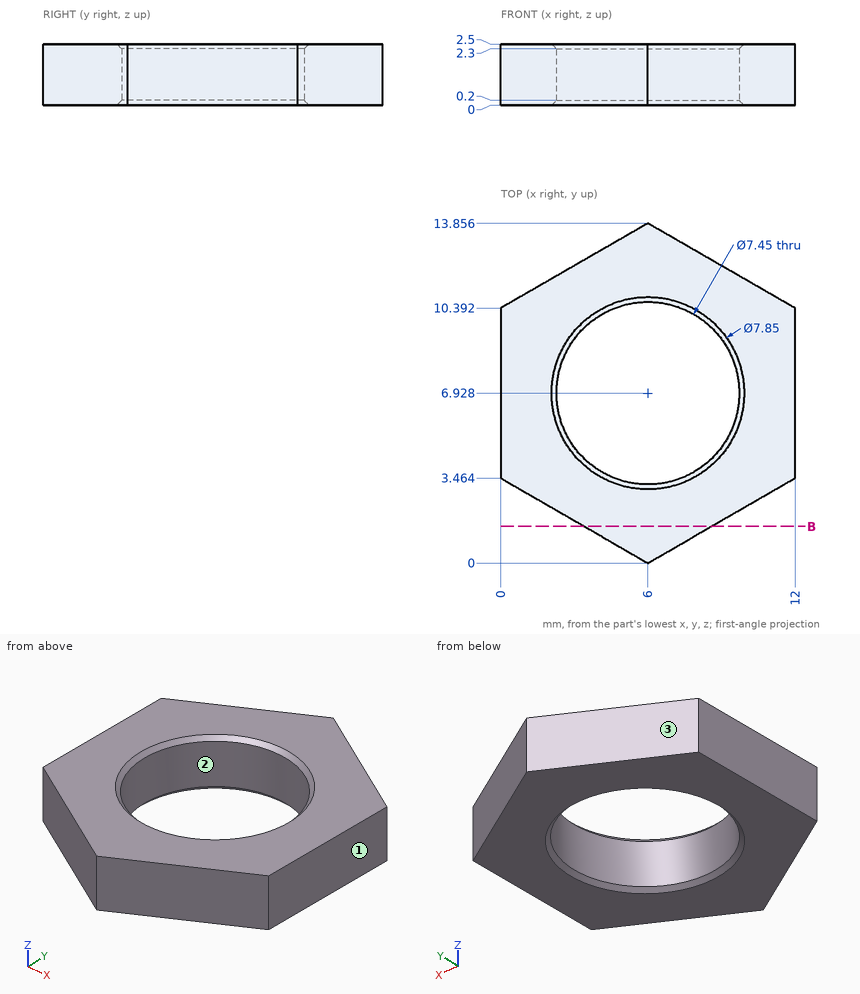
The figure shows three views and two pictorial views of one solid part (mm, origin at its lowest corner). Answer the questions. Round coordinates to 2 decimals unless told otherwise and drop trailing zeros. Order: outer loops, then holes, each group sorted by start corner. A loop starts at its lowest first (then second) coordinate and runs counter-clockwise, first axis right, second up. Notation, with made-up numbers: M 54,-18 L 76,-18 A13 ccw 76,4 Z; hole C 85,-5 d3. An arc over 180 degrees is marked long. Put each result on its own line as item: value. Start each with the question number.
Q1. A flat-ended cylindrical pin translates along its axis: pin 1 (4.5 mm diameter, centred on x = 6, y = 6.93, fed in from +Z). Find the tip coordinate at first contact, or state that the pin passes through.
Q2. Section B-B, the plane y = 1.5 is taken. Write down the section's boundary in (x, z).
Q3. Straight lines are drawn through the part: L1, parallel to X at y = 7, z = 1.6 (1 decimal); L2, parallel to Y at x = 6.25, z = 2.05 (1 decimal); L3, parallel to X at y = 9, z = 2.45 (1 decimal). For each, find the intervals that lie inside material, in ascending order. Write a range as [from, to].
Q4. For a pull along X with two mould halves and no side action, classify the marked faces 1, 2 and 3 as pulls with the +X half, pulls with the -X half, needs draft (parallel to the pull), parting line crosses it, or undercut.
Findings below:
1. pin 1: passes through
2. outline: M 3.4,0 L 8.6,0 L 8.6,2.5 L 3.4,2.5 Z
3. L1: x = [0, 2.3], [9.7, 12]
3. L2: y = [0.1, 3.2], [10.6, 13.7]
3. L3: x = [0, 2.7], [9.3, 12]
4. face 1: pulls with the +X half
4. face 2: undercut
4. face 3: pulls with the -X half
